Here's how the part is built. I have some questions about the finished solid (model axes, mm). Face numbers are marked on the shaded views. Round coordinates to 2 decimals unless told otherwise and drop trailing zeros. Write each loop counter-clockwise with the first axis right and the second up, starting at its lowest first coordinate (ties: lowest second). Pieces come first, ordered by that corner, then holes. Notation, with made-up numbers: M -20,47 L 19,47 A26 cw 19,63 Z; hole C 60,76.25 d5. An arc over 180 degrees is marked long. Use one line per item in the form item = value. Start each with the question number.
Q1. I want a section at A-A on y = 14.75. List the corners of the cut face in (x, z) for me, and give its area (3 significant figures).
Q2. I need wall thicknesses on line 1 along X through (y, z) = (12.5, 0); line 2 along Z through (x, y) = (0, 10.5); line 3 along X through (y, z) = (3.45, 0). Which ranges of each line are inside material? Lowest first, please. Write a range as from..to.
Q3. I'm going to push flat-ended pins straight in: pin 1 Ø4 at (y, z) = (4, 5) entering from -X; pin 2 Ø5.5 at (x, z) = (0, 0) entering from -Y; pin 3 Ø2 at (x, y) = (-0.5, 3.5) entering from +Z. Where does each tip first touch, or does it pass through?
Q4. We'd pull the mould along Z, two halves only. Please class the marked faces 1, 2 and 3: +Z half, -Z half, draft (parallel to the pull), parting line (faces both ways), or undercut.
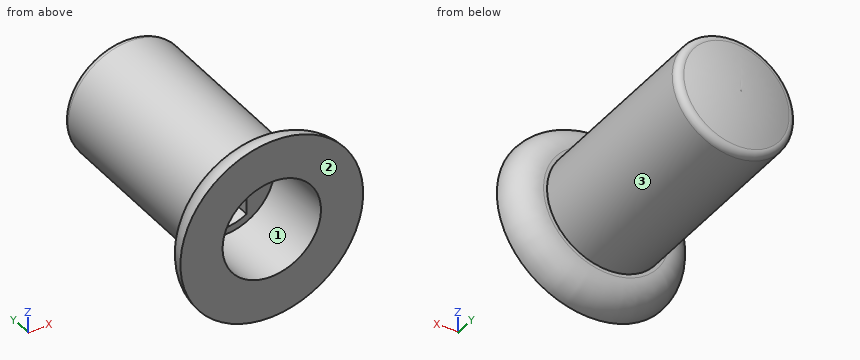
```python
from build123d import *

# Parameters (mm, degrees)
SKETCH1_R           = 4.25
BOSS_EXTRUDE1_DEPTH = 16
FILLET1_R           = 0.5
SKETCH3_R           = 3.75
BOSS_EXTRUDE3_DEPTH = 0.5
FILLET2_R           = 14
SKETCH5_R           = 3.5
CUT_EXTRUDE1_DEPTH  = 5
SKETCH6_R           = 3
CUT_EXTRUDE2_DEPTH  = 10
SKETCH7_W           = 1.5
SKETCH7_H           = 5.196152422
BOSS_EXTRUDE5_DEPTH = 10
SKETCH8_R           = 6.5
BOSS_EXTRUDE6_DEPTH = 2
SKETCH9_R           = 3.5
CUT_EXTRUDE3_DEPTH  = 2
FILLET3_R           = 2


# Some blends are built 0.0001 mm under size
with BuildPart() as part:
    # Sketch1 → Boss-Extrude1 (new body)
    with BuildSketch(Plane(origin=(0, 0, 0), x_dir=(1, 0, 0), z_dir=(0, 1, 0))):
        with Locations(Location((0, 0, 0), (0, 0, 270))):
            Circle(SKETCH1_R)
    extrude(amount=BOSS_EXTRUDE1_DEPTH)

    # Fillet1
    fillet1_edges = [part.edges().sort_by_distance(p)[0] for p in [
        (0, 16, -4.25),
    ]]
    fillet(fillet1_edges, radius=FILLET1_R)

    # Sketch3 → Boss-Extrude3 (add)
    with BuildSketch(Plane(origin=(0, 16, 0), x_dir=(1, 0, 0), z_dir=(0, 1, 0))):
        with Locations(Location((0, 0, 0), (0, 0, 270))):
            Circle(SKETCH3_R)
    extrude(amount=BOSS_EXTRUDE3_DEPTH)

    # Fillet2
    # the kernel refuses this fillet: 14 mm, written as the material it takes off along each edge
    with BuildSketch(Plane(origin=(0, 16.5, 0), x_dir=(0, 0, 1), z_dir=(-1, 0, 0))) as fillet2_piece_1:
        with BuildLine():
            CenterArc((0.041900756, -14), FILLET2_R, 74.641114419, 15.358885581)
            Line((0.041900756, 0), (0.041900756, 0.28))
            Line((0.041900756, 0.28), (3.75, 0.28))
            Line((3.75, 0.28), (4.03, 0))
            ThreePointArc((4.03, 0), (4.03, -0.25), (3.824161985, -0.23))
            Line((3.824161985, -0.23), (3.75, -0.5))
        make_face()
    revolve(axis=Axis((0, 16.5, 0), (0, 1, 0)), mode=Mode.SUBTRACT)

    # Sketch5 → Cut-Extrude1 (cut)
    with BuildSketch(Plane.XZ):
        with Locations(Location((0, 0, 0), (0, 0, 270))):
            Circle(SKETCH5_R)
    extrude(amount=-CUT_EXTRUDE1_DEPTH, mode=Mode.SUBTRACT)

    # Sketch6 → Cut-Extrude2 (cut)
    with BuildSketch(Plane.XZ.offset(-5)):
        with Locations(Location((0, 0, 0), (0, 0, 270))):
            Circle(SKETCH6_R)
    extrude(amount=-CUT_EXTRUDE2_DEPTH, mode=Mode.SUBTRACT)

    # Sketch7 → Boss-Extrude5 (add)
    with BuildSketch(Plane.XZ.offset(-15)):
        with Locations((2.25, 0)):
            Rectangle(SKETCH7_W, SKETCH7_H)
    extrude(amount=BOSS_EXTRUDE5_DEPTH)

    # Sketch8 → Boss-Extrude6 (add)
    with BuildSketch(Plane.XZ):
        with Locations(Location((0, 0, 0), (0, 0, 270))):
            Circle(SKETCH8_R)
    extrude(amount=-BOSS_EXTRUDE6_DEPTH)

    # Sketch9 → Cut-Extrude3 (cut)
    with BuildSketch(Plane.XZ):
        with Locations(Location((0, 0, 0), (0, 0, 270))):
            Circle(SKETCH9_R)
    extrude(amount=-CUT_EXTRUDE3_DEPTH, mode=Mode.SUBTRACT)

    # Fillet3
    fillet3_edges = [part.edges().sort_by_distance(p)[0] for p in [
        (0, 2, 6.5),
    ]]
    fillet(fillet3_edges, radius=FILLET3_R - 0.0001)  # a hair under: the kernel refuses the full size


solid = part.part
```
Reported:
q1.outline = C 0,0 d8.5; hole M 1.5,-2.6 L 1.5,2.6 A3 ccw long Z
q1.area = 34.0 mm^2
q2.line_1 = -4.25..-3, 1.5..4.25
q2.line_2 = -4.25..-3, 3..4.25
q2.line_3 = -4.25..-3.5, 3.5..4.25
q3.pin_1 = -3.01
q3.pin_2 = 5
q3.pin_3 = 4.25
q4.face_1 = undercut
q4.face_2 = draft
q4.face_3 = parting line
